from build123d import *

# Parameters (mm, degrees)
F1_DEPTH = 6
F2_D     = 25
F3_D     = 25
F4_D     = 25


with BuildPart() as f1:
    # F0 (on Top) → F1 (new body)
    with BuildSketch(Plane.XY):
        with BuildLine():
            Line((-275, -150), (275, -150))
            ThreePointArc((275, -150), (292.67767, -142.67767), (300, -125))
            Line((300, -125), (300, 125))
            ThreePointArc((300, 125), (292.67767, 142.67767), (275, 150))
            Line((275, 150), (-275, 150))
            ThreePointArc((-275, 150), (-292.67767, 142.67767), (-300, 125))
            Line((-300, 125), (-300, -125))
            ThreePointArc((-300, -125), (-292.67767, -142.67767), (-275, -150))
        make_face()
    extrude(amount=F1_DEPTH)

    # F2 (through all)
    with Locations(Plane(origin=(0, 0, 0), x_dir=(1, 0, 0), z_dir=(0, 0, -1))):
        with Locations((-275, -125)):
            Hole(F2_D / 2)

    # F3 (through all)
    with Locations(Plane(origin=(0, 0, 0), x_dir=(1, 0, 0), z_dir=(0, 0, -1))):
        with Locations((-275, 125), (275, -125)):
            Hole(F3_D / 2)

    # F4 (through all)
    with Locations(Plane(origin=(0, 0, 0), x_dir=(1, 0, 0), z_dir=(0, 0, -1))):
        with Locations((275, 125)):
            Hole(F4_D / 2)


solid = f1.part
CAD build for the part. Positions are in the model's coordinates, mm. Coordinates: 2 decimals unless noted, no trailing zeros.
Item 1: Pin check, flat tip, straight feed: pin 1 Ø2 at (x, y) = (86.5, 33) entering from -Z. Stop position of the tip, or through.
Check sheet entries:
pin 1: stops at z = 0
Item 2: Two-plate mould, pull along Y, no slides. Class faces 1 (the face through (-4, 2, 0)), 2 (the face through (-286.923, -128.755, 3.042)), 3 (the face through (-292.482, 142.871, 2.958)): +Y half, -Y half, draft (parallel to the pull), parting line (faces both ways), or undercut.
Check sheet entries:
face 1: draft
face 2: undercut
face 3: +Y half
Item 3: Drill centre lines: L1, parallel to X at y = -125, z = 4.4; L2, parallel to Y at x = -275, z = 2.15; L3, parallel to Y at x = -268.5, z = 1.7. Where is each one in solid material? Low to high.
Check sheet entries:
L1: x = -300 to -287.5, -262.5 to 262.5, 287.5 to 300
L2: y = -150 to -137.5, -112.5 to 112.5, 137.5 to 150
L3: y = -150 to -135.68, -114.32 to 114.32, 135.68 to 150
